Input: dimensioned drawing with shaded views. Units: mm. Origin: part minimum x, y, z. Round coordinates to 2 decimals unless told otherwise and drop trailing zeros. Order: outer loops, then holes, each group sorted by start corner. A loop starts at its lowest first (then second) coordinate and runs counter-clockwise, first axis right, second up. Notation, with made-up numbers: (-8, 82.5) -> (24, 82.5) arc R18 ccw to (24, 107.5) -> close; hole circle Ø5 at (77.5, 53). An arc over 180 degrees is marked (long way). Use a Markdown table: item, result. Add a question column.
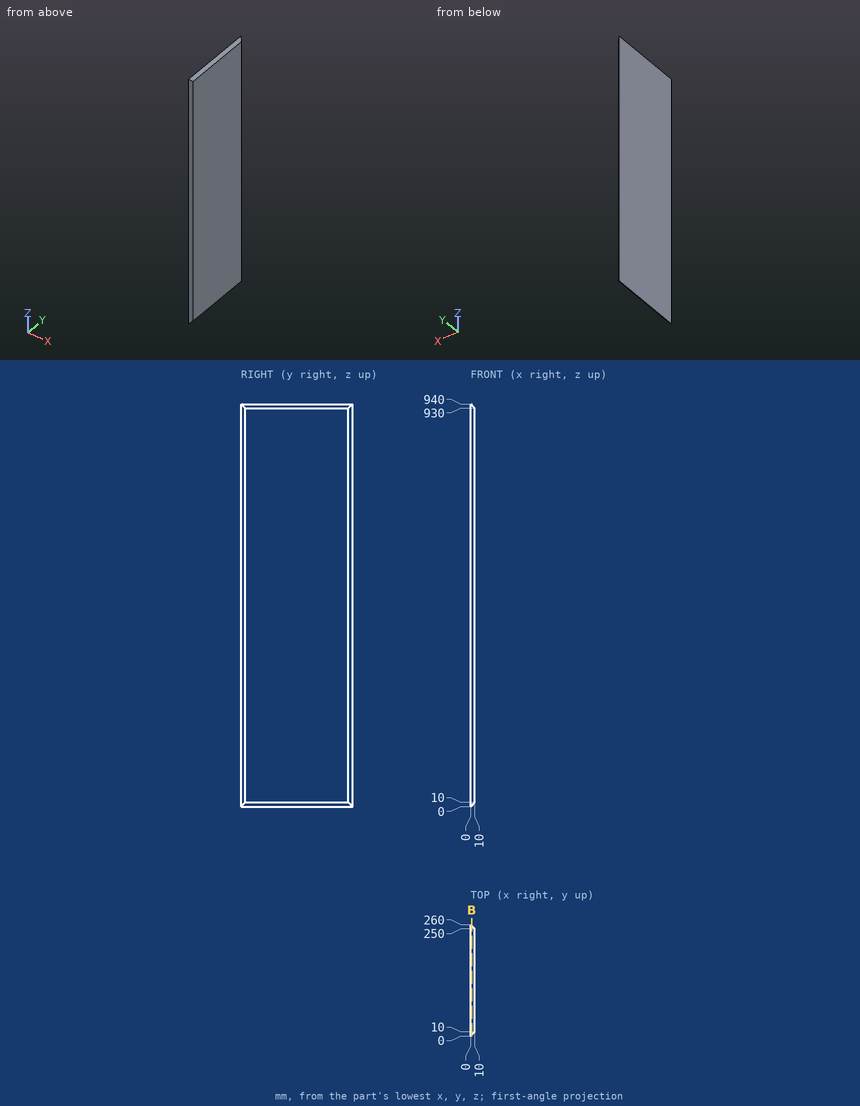
1) Line query: probe 1 along Z at (x, y) = (4.5, 38); probe 2 along Y at (x, z) = (2.75, 538.5); probe 3 along Y at (x, z) = (2.5, 331). Output: solid intervals per line, ascending. Write a range as from..to.
2) Section B-B on x = 2.75. Output: boundary loops of the cut face in (y, z), then the cut area to 3 significant figures.
3) First-contact query: pin 1 Ø5 at (x, z) = (7, 361.5) entering from -Y; pin 2 Ø4 at (x, z) = (1, 301) entering from +Y; pin 3 Ø1.5 at (x, z) = (3, 311) entering from +Y. Flat tips, straight axial feed; report the tip coordinate or a pass-through.
Conclusion:
| question | item | result |
|---|---|---|
| 1 | probe 1 | z = 4.5..935.5 |
| 1 | probe 2 | y = 2.75..257.25 |
| 1 | probe 3 | y = 2.5..257.5 |
| 2 | outline | (2.75, 2.75) -> (257.25, 2.75) -> (257.25, 937.25) -> (2.75, 937.25) -> close |
| 2 | area | 238,000 mm^2 |
| 3 | pin 1 | stops at y = 4.5 |
| 3 | pin 2 | stops at y = 260 |
| 3 | pin 3 | stops at y = 257.75 |
